The model under review builds one solid part; all positions refer to its coordinate system, in mm. A direction names the side the tool comes from. Give positions to 0.01 mm unless a question says otherwise; leave off trailing zeros. Loops run counter-clockwise (first coordinate to the right, second up) from the corner with the lowest first, then second, coordinate; pieces in that order, holes last. Notation, with made-up numbers: (6, 36) - (22, 36) arc R18 cw to (22, 40) - close; hole circle Ø6 at (-37.75, 11.25). An arc over 180 degrees is marked (long way). Return JSON: item names as keys, results as strings. Group by question number.
```python
from build123d import *

# Parameters (mm, degrees)
SKETCH2_W           = 63.3
SKETCH2_H           = 30.32
BOSS_EXTRUDE1_DEPTH = 5
SKETCH1_R           = 1.5
SKETCH1_W           = 40.64
SKETCH1_H           = 20.32
CUT_EXTRUDE7_DEPTH  = 6
FILLET1_R           = 2
SKETCH4_W           = 5.3
SKETCH4_H           = 1.27
CUT_EXTRUDE8_DEPTH  = 6
SKETCH5_W           = 5.3
SKETCH5_H           = 1.27
CUT_EXTRUDE9_DEPTH  = 6


with BuildPart() as part:
    # Sketch2 → Boss-Extrude1 (new body)
    with BuildSketch(Plane(origin=(0, 0, 0), x_dir=(0, 0, -1), z_dir=(1, 0, 0))):
        Rectangle(SKETCH2_W, SKETCH2_H)
        Polygon((181.65, 5), (31.65, 5), (31.65, 0), (31.65, -5), (181.65, -5), (181.65, 0), align=None)
        Polygon((181.65, 15.16), (181.65, 5), (181.65, 0), (181.65, -5), (181.65, -15.16), (244.95, -15.16), (244.95, 15.16), align=None)
    extrude(amount=BOSS_EXTRUDE1_DEPTH)

    # Sketch1 → Cut-Extrude7 (cut, through all)
    with BuildSketch(Plane(origin=(0, 0, 0), x_dir=(0, 0, -1), z_dir=(1, 0, 0))):
        with Locations((-24.13, 5.08)):
            Circle(SKETCH1_R)
        with Locations((-24.13, -5.08)):
            Circle(SKETCH1_R)
        with Locations((24.13, 5.08)):
            Circle(SKETCH1_R)
        with Locations((24.13, -5.08)):
            Circle(SKETCH1_R)
        with Locations((189.17, -5.08)):
            Circle(SKETCH1_R)
        with Locations((189.17, 5.08)):
            Circle(SKETCH1_R)
        with Locations((237.43, -5.08)):
            Circle(SKETCH1_R)
        with Locations((237.43, 5.08)):
            Circle(SKETCH1_R)
        Rectangle(SKETCH1_W, SKETCH1_H)
        with Locations((213.3, 0)):
            Rectangle(SKETCH1_W, SKETCH1_H)
    extrude(amount=CUT_EXTRUDE7_DEPTH, mode=Mode.SUBTRACT)

    # Fillet1
    fillet1_edges = [part.edges().sort_by_distance(p)[0] for p in [
        (2.5, 5, -31.65),
        (2.5, 5, -181.65),
        (2.5, 15.16, -181.65),
        (2.5, 15.16, -244.95),
        (2.5, -15.16, -244.95),
        (2.5, -15.16, -181.65),
        (2.5, -5, -181.65),
        (2.5, -5, -31.65),
        (2.5, -15.16, -31.65),
        (2.5, -15.16, 31.65),
        (2.5, 15.16, 31.65),
        (2.5, 15.16, -31.65),
    ]]
    fillet(fillet1_edges, radius=FILLET1_R)

    # Sketch4 → Cut-Extrude8 (cut, through all)
    with BuildSketch(Plane(origin=(5, 0, 0), x_dir=(0, 0, -1), z_dir=(1, 0, 0))):
        with Locations((-22.97, 0)):
            Rectangle(SKETCH4_W, SKETCH4_H)
        with Locations((22.97, 0)):
            Rectangle(SKETCH4_W, SKETCH4_H)
    extrude(amount=-CUT_EXTRUDE8_DEPTH, mode=Mode.SUBTRACT)

    # Sketch5 → Cut-Extrude9 (cut, through all)
    with BuildSketch(Plane(origin=(5, 0, 0), x_dir=(0, 0, -1), z_dir=(1, 0, 0))):
        with Locations((236.27, 0)):
            Rectangle(SKETCH5_W, SKETCH5_H)
        with Locations((190.33, 0)):
            Rectangle(SKETCH5_W, SKETCH5_H)
    extrude(amount=-CUT_EXTRUDE9_DEPTH, mode=Mode.SUBTRACT)


solid = part.part
```
1) We need section C-C, the plane z = -169. Write out the cut boundary in (x, y), plus the area to 3 significant figures.
2) We need section B-B, the plane x = 3.95. Count the separate pieces of the cut face and the enclosed holes in it, plus the area to 3 significant figures.
3) Draft analysis for pull direction Z (two halves, no side actions). For faces 1 (the face through (2, 0, 31.65)), 2 (the face through (2, 0, -244.95)), 3 (the face through (2, 10.16, 0)), 4 (the face through (2, -15.16, 0)), state which applies: +Z half, -Z half, draft (parallel to the pull), parting line (faces both ways), or undercut.
4) For pin 1 Ø1.5 at (x, z) = (1.5, -114.5) entering from -Y, flat-tipped, find the tip position at first contact; note if it passes through.
5) Tool access review of faces 5 (the face through (2, -5, -106)), 6 (the face through (2, 5, -108)), 7 (the face through (3, -0.635, 23)), 8 (the face through (0, 1, -106)): name each direction out of +Z, -Z, +X, -X, +Y, -Y from which nothing blocks a thin tool from reaching the whole face with its end or side.
6) To check wall thickness, follow line 1 (Y direction, x = 3.15, z = -237.43) (3 decimals); line 2 (Z direction, x = 4.8, y = -9.5); line 3 (Z direction, x = 4.3, y = 0). State the ranges of each line that lie inside material, in increasing order.
7) We need section A-A, the plane z = -220.5. Write out the cut boundary in (x, y).
Findings:
{
 "1": {"outline": "(0, -5) - (5, -5) - (5, 5) - (0, 5) - close", "area": "50.0 mm^2"},
 "2": {"separate pieces": "1", "enclosed holes": "10", "area": "3,600 mm^2"},
 "3": {"face 1": "+Z half", "face 2": "-Z half", "face 3": "undercut", "face 4": "draft"},
 "4": {"pin 1": "stops at y = -5"},
 "5": {"face 5": "+X, -X, -Y", "face 6": "+X, -X, +Y", "face 7": "+X, -X", "face 8": "+Z, -Z, -X, +Y, -Y"},
 "6": {"line 1": "y = -15.16 to -6.58, -3.58 to -0.635, 0.635 to 3.58, 6.58 to 15.16", "line 2": "z = -244.95 to -233.62, -192.98 to -181.65, -31.65 to -20.32, 20.32 to 31.65", "line 3": "z = -244.95 to -238.92, -187.68 to -25.62, 25.62 to 31.65"},
 "7": {"outline": "(0, -15.16) - (5, -15.16) - (5, -10.16) - (0, -10.16) - close; (0, 10.16) - (5, 10.16) - (5, 15.16) - (0, 15.16) - close"}
}
